CAD build for the part. Positions are in the model's coordinates, mm. Face numbers are marked on the shaded views. A direction names the side the tool comes from. Coordinates: 2 decimals unless noted, no trailing zeros. Order: outer loops, then holes, each group sorted by start corner. A loop starts at its lowest first (then second) coordinate and runs counter-clockwise, first axis right, second up. Notation, with made-up numbers: M 5,88.5 L 36,88.5 A26 ccw 36,123.5 Z; hole C -10,-19 d11. An arc over 180 degrees is marked long. One line per item, written item: value.
from build123d import *

# Parameters (mm, degrees)
BOSS_EXTRUDE2_DEPTH = 38.1
SKETCH5_W           = 20.4724
SKETCH5_H           = 40.64
CUT_EXTRUDE2_DEPTH  = 154.893000964
CIRPATTERN1_COUNT   = 5
SKETCH6_R           = 10.680701414
CUT_EXTRUDE3_DEPTH  = 154.893000964


with BuildPart() as part:
    # Sketch4 → Boss-Extrude2 (new body)
    with BuildSketch(Plane(origin=(0, 0, 0), x_dir=(1, 0, 0), z_dir=(0, 1, 0))):
        Polygon((-102.747316485, 33.402541556), (0, 108.048298), (102.743, 33.396600424), (63.494349621, -87.38644244), (-63.505650326, -87.382770618), align=None)
    extrude(amount=BOSS_EXTRUDE2_DEPTH)

    # Sketch5 → Cut-Extrude2 (cut, through all)
    with BuildSketch(Plane(origin=(0, 38.1, 0), x_dir=(1, 0, 0), z_dir=(0, 1, 0))):
        with Locations((0.019749621, -60.714607261)):
            Rectangle(SKETCH5_W, SKETCH5_H)
    cut_extrude2 = extrude(amount=-CUT_EXTRUDE2_DEPTH, mode=Mode.SUBTRACT)

    # CirPattern1: Cut-Extrude2 ×5 about axis
    cirpattern1_axis = Axis((0, 0, 0), (0, 1, 0))
    for i in range(1, CIRPATTERN1_COUNT):
        add(cut_extrude2.rotate(cirpattern1_axis, i * 360 / CIRPATTERN1_COUNT), mode=Mode.SUBTRACT)

    # Sketch6 → Cut-Extrude3 (cut, through all)
    with BuildSketch(Plane.XZ):
        with Locations(Location((0, 0, 0), (0, 0, 270))):
            Circle(SKETCH6_R)
    extrude(amount=-CUT_EXTRUDE3_DEPTH, mode=Mode.SUBTRACT)


solid = part.part
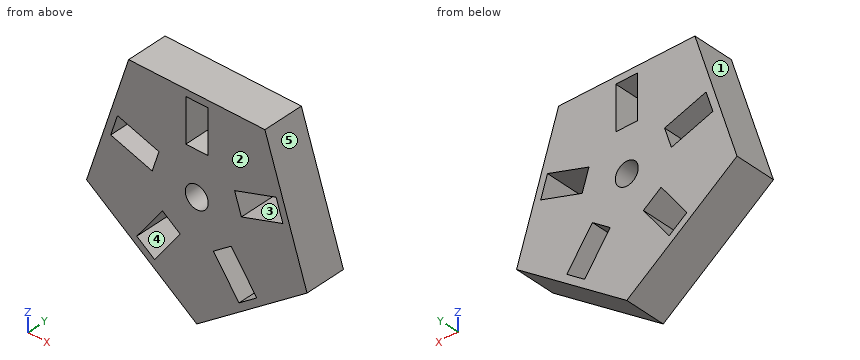
Q1. Which spindle directions (+Z, -Z, +X, -X, +Y, -Y) get a long thin tool onto all of the face, cutting with end or side? Do the marked faces 4 and 5. Say none if no direction does.
Recorded:
face 4: +Y, -Y
face 5: +Z, +X, +Y, -Y
Q2. Drill centre lines: line 1 along Z through (x, y) = (54, 26); line 2 along Z through (x, y) = (2, 16.5); line 3 along X through (y, z) = (19, 0). Where is each one in solid material? Low to high.
Recorded:
line 1: z = -68.81 to -60.93, -56.94 to 6.76, 28.29 to 87.39
line 2: z = -106.6 to -10.49, 10.49 to 40.39, 81.03 to 87.38
line 3: x = -91.9 to -10.68, 10.68 to 91.89
Q3. Mould opens along Z. For the marked faces 1, 2 and 3 say: released by +Z, released by -Z, zero draft, split by the parting line, or undercut.
Recorded:
face 1: released by +Z
face 2: zero draft
face 3: undercut
Q4. Slice it at D-D (z = -45). List the corners of the cut face in (x, y), plus the area to 3 significant figures.
Recorded:
outline: M -86.78,0 L -45.37,0 L -45.37,38.1 L -86.78,38.1 Z; M -20.07,0 L 20.02,0 L 20.02,38.1 L -20.07,38.1 Z; M 45.32,0 L 86.77,0 L 86.77,38.1 L 45.32,38.1 Z
area: 4,680 mm^2
Q5. Pin check, flat tips, straight feed: pin 1 Ø19 at (y, z) = (22.5, 61.5) entering from +X; pin 2 Ø2 at (x, y) = (46, 34) entering from -Z; pin 3 Ø12 at (y, z) = (21.5, 64.5) entering from -X. Stop position of each tip, or through.
Recorded:
pin 1: stops at x = 74.99
pin 2: stops at z = -75.35
pin 3: stops at x = -72.89
Q6. Slice it at C-C (x = -58.5). List the corners of the cut face in (y, z).
Recorded:
outline: M 0,-65.55 L 38.1,-65.55 L 38.1,8.27 L 0,8.27 Z; M 0,29.79 L 38.1,29.79 L 38.1,87.38 L 0,87.38 Z
Q7. Slice it at A-A (y = 18.5). List the corners of the cut face in (x, z) (1 decimal).
Recorded:
outline: M -102.7,-33.4 L 0,-108 L 102.7,-33.4 L 63.5,87.4 L -63.5,87.4 Z; hole M -80.2,15.3 L -41.6,2.8 L -35.2,22.2 L -73.9,34.8 Z; hole M -55.9,-59.5 L -39.4,-71.6 L -15.5,-38.7 L -32,-26.7 Z; hole C 0,0 d21.4; hole M -10.2,40.4 L 10.3,40.4 L 10.3,81 L -10.2,81 Z; hole M 15.4,-38.7 L 39.3,-71.6 L 55.9,-59.6 L 32,-26.7 Z; hole M 35.3,22.2 L 41.6,2.7 L 80.2,15.3 L 73.9,34.8 Z
Q8. Slice it at B-B (z = 0). List the corners of the cut face in (x, y).
Recorded:
outline: M -91.9,0 L -10.68,0 L -10.68,38.1 L -91.9,38.1 Z; M 10.68,0 L 91.89,0 L 91.89,38.1 L 10.68,38.1 Z
